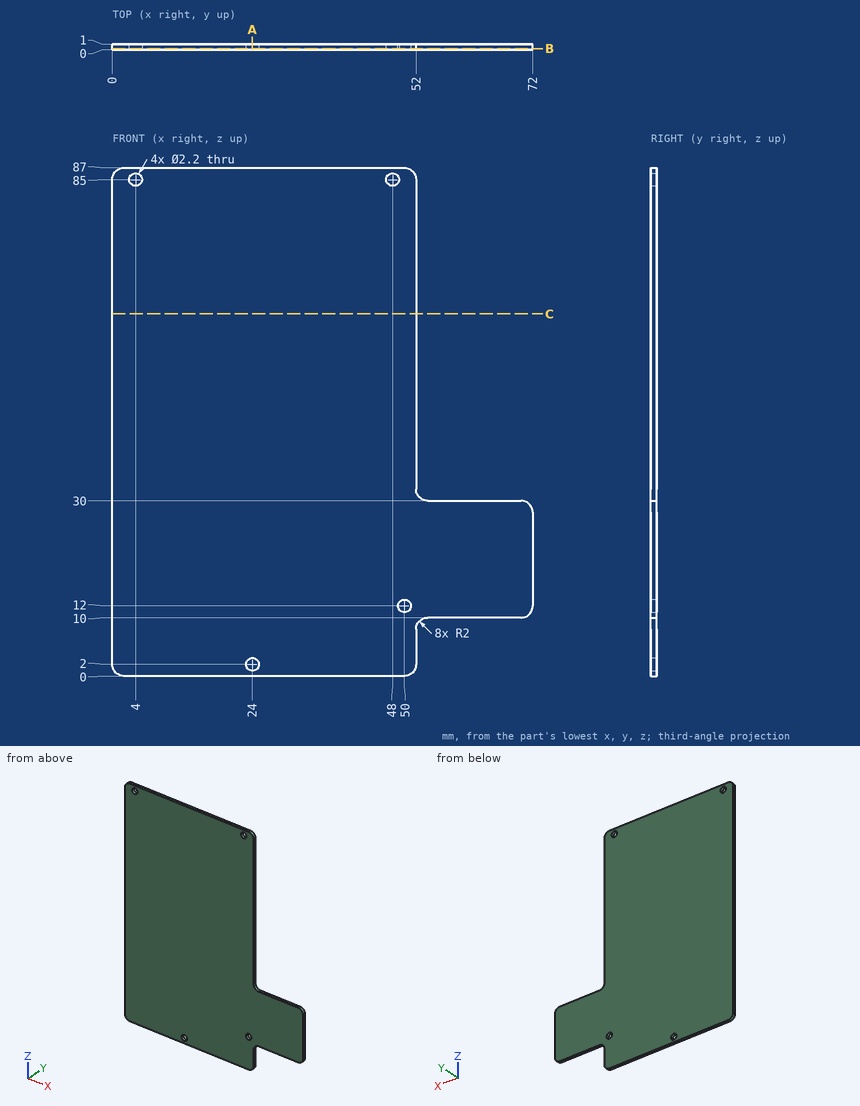
Check sheet for the drawn part. Datum: minimum x, y, z corner. Units: mm. Give positions to 0.01 mm unless a question says otherwise; leave off trailing zeros. Write each loop counter-clockwise with the first axis right and the second up, starting at its lowest first coordinate (ties: lowest second). Pieces come first, ordered by that corner, then holes.
(1) Cross-section at A-A (x = 24). Enter the section's corners in (y, z), plus the area to 3 significant figures.
(2) Material ranges on line 1 (X direction, y = 0.8, z = 85); line 2 (X direction, y = 0.35, z = 12); line 3 (Z direction, x = 50, y = 0.7), recorded low to high.
(3) Cross-section at C-C (z = 62). Enter the section's corners in (x, y), plus the area to 3 significant figures.
(4) Cross-section at B-B (y = 0.2). Enter the section's corners in (x, z).
(5) Gauge pin test, flat ends, axial feed: pin 1 (3.5 mm diameter, centred on x = 24, z = 2, fed in from -Y); pin 2 (0.5 mm diameter, centred on x = 59, y = 0.5, fed in from +Z). Record the tip position at first contact, or that the pin passes through.
Worked out:
1. outline: (0, 0) - (1, 0) - (1, 0.9) - (0, 0.9) - close; (0, 3.1) - (1, 3.1) - (1, 87) - (0, 87) - close
1. area: 84.8 mm2
2. line 1: x = 0 to 2.9, 5.1 to 46.9, 49.1 to 52
2. line 2: x = 0 to 48.9, 51.1 to 72
2. line 3: z = 0 to 10.9, 13.1 to 87
3. outline: (0, 0) - (52, 0) - (52, 1) - (0, 1) - close
3. area: 52.0 mm2
4. outline: (0, 2) arc R2 ccw to (2, 0) - (50, 0) arc R2 ccw to (52, 2) - (52, 8) arc R2 cw to (54, 10) - (70, 10) arc R2 ccw to (72, 12) - (72, 28) arc R2 ccw to (70, 30) - (54, 30) arc R2 cw to (52, 32) - (52, 85) arc R2 ccw to (50, 87) - (2, 87) arc R2 ccw to (0, 85) - close; hole circle Ø2.2 at (4, 85); hole circle Ø2.2 at (24, 2); hole circle Ø2.2 at (48, 85); hole circle Ø2.2 at (50, 12)
5. pin 1: stops at y = 0
5. pin 2: stops at z = 30
